Design review of the part built by this model. Coordinates are the model's own, in mm. Round coordinates to 2 decimals unless told otherwise and drop trailing zeros. Order: outer loops, then holes, each group sorted by start corner. A loop starts at its lowest first (then second) coordinate and runs counter-clockwise, first axis right, second up. Notation, with made-up numbers: M 63,-21.5 L 122,-21.5 A30 cw 122,6.5 Z; hole C 38,88.5 d5. An arc over 180 degrees is marked long. Write each question's results on one line, items separated by ' | '. Start each with the question number.
Item 1: Take a section at A-A, the plane x = 180. Write out the cut boundary in (y, z) (3 decimals), plus the area to 3 significant figures.
Item 2: Wall thickness on line 1 (Z direction, x = 56, y = 2.8); line 2 (Z direction, x = 152.5, y = 2.2): over which ranges is each line inside the solid? List them lowest first. Write a range as [from, to].
Item 3: Take a section at B-B, the plane y = 1.5. Count the separate pieces of the cut face and the enclosed holes in it, plus the area to 3 significant figures.
Item 4: Clearance check with a flat-ended pin moving along its axis: pin 1 (2 mm diameter, centred on x = 84, z = -10.5, fed in from -Y). State where the tip first meets the part, or that it passes through.
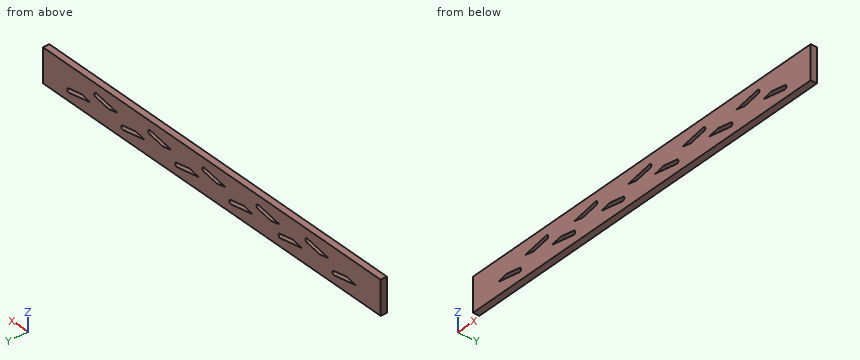
```python
from build123d import *

# Parameters (mm, degrees)
SKETCH4_W           = 200
SKETCH4_H           = 17.1
BOSS_EXTRUDE2_DEPTH = 3.175
CUT_EXTRUDE3_DEPTH  = 3.175


with BuildPart() as part:
    # Sketch4 → Boss-Extrude2 (new body)
    with BuildSketch(Plane(origin=(0, 0, 0), x_dir=(1, 0, 0), z_dir=(0, 1, 0))):
        with Locations((100, 8.55)):
            Rectangle(SKETCH4_W, SKETCH4_H)
    extrude(amount=BOSS_EXTRUDE2_DEPTH)

    # Sketch5 → Cut-Extrude3 (cut)
    with BuildSketch(Plane(origin=(0, 3.175, 0), x_dir=(1, 0, 0), z_dir=(0, 1, 0))):
        with BuildLine():
            ThreePointArc((59.356356651, 13.033114886), (60.52246094, 12.232989403), (59.722335457, 11.066885114))
            Line((59.722335457, 11.066885114), (51.857416371, 9.602969892))
            Line((51.857416371, 9.602969892), (46.821641859, 10.7))
            Line((46.821641859, 10.7), (59.356356651, 13.033114886))
        make_face()
        with BuildLine():
            ThreePointArc((72.822542019, 6.383114886), (73.622667502, 5.217010597), (72.456563214, 4.416885114))
            Line((72.456563214, 4.416885114), (59.921848421, 6.75))
            Line((59.921848421, 6.75), (64.957622934, 7.847030108))
            Line((64.957622934, 7.847030108), (72.822542019, 6.383114886))
        make_face()
        with BuildLine():
            ThreePointArc((88.456563214, 13.033114886), (89.622667502, 12.232989403), (88.822542019, 11.066885114))
            Line((88.822542019, 11.066885114), (80.957622934, 9.602969892))
            Line((80.957622934, 9.602969892), (75.921848421, 10.7))
            Line((75.921848421, 10.7), (88.456563214, 13.033114886))
        make_face()
        with BuildLine():
            ThreePointArc((104.822542019, 6.383114886), (105.622667502, 5.217010597), (104.456563214, 4.416885114))
            Line((104.456563214, 4.416885114), (91.921848421, 6.75))
            Line((91.921848421, 6.75), (96.957622934, 7.847030108))
            Line((96.957622934, 7.847030108), (104.822542019, 6.383114886))
        make_face()
        with BuildLine():
            ThreePointArc((120.456563214, 13.033114886), (121.622667502, 12.232989403), (120.822542019, 11.066885114))
            Line((120.822542019, 11.066885114), (112.957622934, 9.602969892))
            Line((112.957622934, 9.602969892), (107.921848421, 10.7))
            Line((107.921848421, 10.7), (120.456563214, 13.033114886))
        make_face()
        with BuildLine():
            ThreePointArc((152.456563214, 13.033114886), (153.622667502, 12.232989403), (152.822542019, 11.066885114))
            Line((152.822542019, 11.066885114), (144.957622934, 9.602969892))
            Line((144.957622934, 9.602969892), (139.921848421, 10.7))
            Line((139.921848421, 10.7), (152.456563214, 13.033114886))
        make_face()
        with BuildLine():
            ThreePointArc((184.456563214, 13.033114886), (185.622667502, 12.232989403), (184.822542019, 11.066885114))
            Line((184.822542019, 11.066885114), (176.957622934, 9.602969892))
            Line((176.957622934, 9.602969892), (171.921848421, 10.7))
            Line((171.921848421, 10.7), (184.456563214, 13.033114886))
        make_face()
        with BuildLine():
            Line((14.821641859, 10.7), (19.857416371, 9.602969892))
            Line((19.857416371, 9.602969892), (27.722335457, 11.066885114))
            ThreePointArc((27.722335457, 11.066885114), (28.52246094, 12.232989403), (27.356356651, 13.033114886))
            Line((27.356356651, 13.033114886), (14.821641859, 10.7))
        make_face()
        with BuildLine():
            Line((35.857416371, 7.847030108), (43.722335457, 6.383114886))
            ThreePointArc((43.722335457, 6.383114886), (44.52246094, 5.217010597), (43.356356651, 4.416885114))
            Line((43.356356651, 4.416885114), (30.821641859, 6.75))
            Line((30.821641859, 6.75), (35.857416371, 7.847030108))
        make_face()
        with BuildLine():
            Line((128.957622934, 7.847030108), (136.822542019, 6.383114886))
            ThreePointArc((136.822542019, 6.383114886), (137.622667502, 5.217010597), (136.456563214, 4.416885114))
            Line((136.456563214, 4.416885114), (123.921848421, 6.75))
            Line((123.921848421, 6.75), (128.957622934, 7.847030108))
        make_face()
        with BuildLine():
            Line((155.921848421, 6.75), (168.456563214, 4.416885114))
            ThreePointArc((168.456563214, 4.416885114), (169.622667502, 5.217010597), (168.822542019, 6.383114886))
            Line((168.822542019, 6.383114886), (160.957622934, 7.847030108))
            Line((160.957622934, 7.847030108), (155.921848421, 6.75))
        make_face()
    extrude(amount=-CUT_EXTRUDE3_DEPTH, mode=Mode.SUBTRACT)


solid = part.part
```
Results list:
1) outline: M 0,-17.1 L 3.175,-17.1 L 3.175,-12.204 L 0,-12.204 Z; M 0,-10.169 L 3.175,-10.169 L 3.175,0 L 0,0 Z | area: 47.8 mm²
2) line 1: [-17.1, -12.41], [-10.37, 0] | line 2: [-17.1, -13.04], [-11.01, 0]
3) separate pieces: 1 | enclosed holes: 11 | area: 3,170 mm²
4) pin 1: y = 0
